Input: part model. Units: mm. Frame: model coordinates. Round coordinates to 2 decimals unless told otherwise and drop trailing zeros. Loops run counter-clockwise (first coordinate to the right, second up) from the corner with the lowest first, then second, coordinate; pieces in that order, holes last.
1) Section D-D, the plane z = -12. Return loops of the section in (x, y).
2) Ray query, line 1 along Y through (x, z) = (0.6, -5.25); line 2 along Z through (x, y) = (2, -43.8); line 3 along Z through (x, y) = (1.3, -41.5). Return the intervals inside material, ascending.
3) Section C-C, the plane z = -5.25. Return loops of the section in (x, y).
4) Section B-B, the plane x = 1.6. Return loops of the section in (y, z).
5) Section A-A, the plane z = -22.75. Return loops of the section in (x, y).
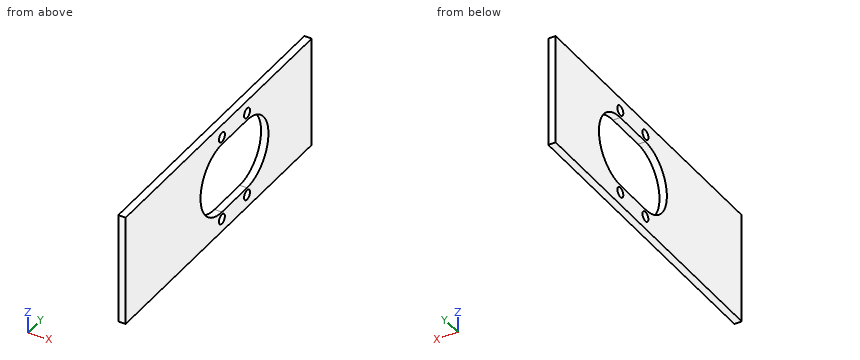
from build123d import *

# Parameters (mm, degrees)
SKETCH1_W           = 45.5
SKETCH1_H           = 126
SKETCH1_R           = 2
BOSS_EXTRUDE1_DEPTH = 3


with BuildPart() as part:
    # Sketch1 → Boss-Extrude1 (new body)
    with BuildSketch(Plane(origin=(0, 0, 0), x_dir=(0, 0, -1), z_dir=(1, 0, 0))):
        with Locations((22.75, -63)):
            Rectangle(SKETCH1_W, SKETCH1_H)
        with Locations((5.25, -60.8)):
            Circle(SKETCH1_R, mode=Mode.SUBTRACT)
        with Locations((40.25, -60.8)):
            Circle(SKETCH1_R, mode=Mode.SUBTRACT)
        with Locations(Location((40.25, -43.8, 0), (0, 0, 180))):
            Circle(SKETCH1_R, mode=Mode.SUBTRACT)
        with Locations(Location((5.25, -43.8, 0), (0, 0, 180))):
            Circle(SKETCH1_R, mode=Mode.SUBTRACT)
        with BuildLine():
            Line((8.25, -60.8), (8.25, -43.8))
            ThreePointArc((8.25, -43.8), (22.75, -29.3), (37.25, -43.8))
            Line((37.25, -43.8), (37.25, -60.8))
            ThreePointArc((37.25, -60.8), (22.75, -75.3), (8.25, -60.8))
        make_face(mode=Mode.SUBTRACT)
    extrude(amount=BOSS_EXTRUDE1_DEPTH)


solid = part.part
Final values:
1. outline: (0, -126) - (3, -126) - (3, -70.53) - (0, -70.53) - close; (0, -34.07) - (3, -34.07) - (3, 0) - (0, 0) - close
2. line 1: y = -126 to -62.8, -58.8 to -45.8, -41.8 to 0
2. line 2: z = -45.5 to -42.25, -38.25 to -37.25, -8.25 to -7.25, -3.25 to 0
2. line 3: z = -45.5 to -37.07, -8.43 to 0
3. outline: (0, -126) - (3, -126) - (3, -62.8) - (0, -62.8) - close; (0, -58.8) - (3, -58.8) - (3, -45.8) - (0, -45.8) - close; (0, -41.8) - (3, -41.8) - (3, 0) - (0, 0) - close
4. outline: (-126, -45.5) - (0, -45.5) - (0, 0) - (-126, 0) - close; hole circle Ø4 at (-60.8, -40.25); hole circle Ø4 at (-60.8, -5.25); hole (-60.8, -37.25) - (-43.8, -37.25) arc R14.5 ccw to (-43.8, -8.25) - (-60.8, -8.25) arc R14.5 ccw to start; hole circle Ø4 at (-43.8, -40.25); hole circle Ø4 at (-43.8, -5.25)
5. outline: (0, -126) - (3, -126) - (3, -75.3) - (0, -75.3) - close; (0, -29.3) - (3, -29.3) - (3, 0) - (0, 0) - close
